from build123d import *

# Parameters (mm, degrees)
ESQUISSE2_W             = 7.209705372
ESQUISSE2_H             = 2.76140959
ENL_V_MAT_EXTRU_1_DEPTH = 7


with BuildPart() as part:
    # Esquisse1 → Révolution1 (revolve)
    with BuildSketch(Plane.XY, mode=Mode.PRIVATE) as r_volution1_sk:
        Polygon((0, 0), (0, 2), (1, 3), (29.26, 3), (29.26, 2.5), (30, 2.5), (30, 3), (44, 3), (45, 2), (45, 0), align=None)
    revolve(r_volution1_sk.sketch.rotate(Axis((-55.939428076, 0, 0), (1, 0, 0)), 90), axis=Axis((-55.939428076, 0, 0), (1, 0, 0)))  # turned: the seam where the file's is

    # Esquisse2 → Enlèv. mat.-Extru.1 (cut)
    with BuildSketch(Plane(origin=(45, 0, 0), x_dir=(0, 0, -1), z_dir=(1, 0, 0))):
        with Locations((-0.271519353, 2.880704795)):
            Rectangle(ESQUISSE2_W, ESQUISSE2_H)
    extrude(amount=-ENL_V_MAT_EXTRU_1_DEPTH, mode=Mode.SUBTRACT)


solid = part.part
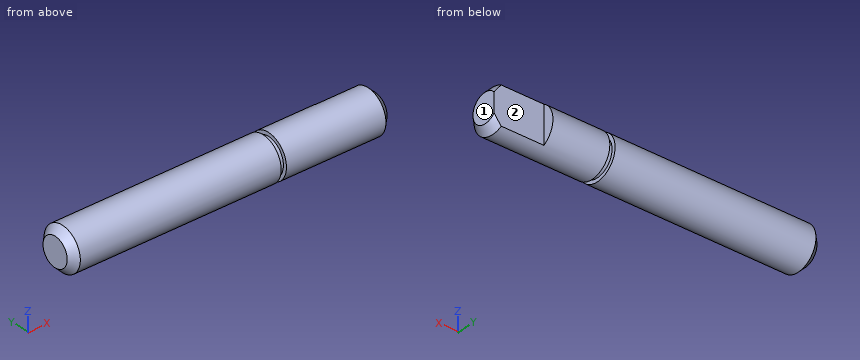
Build history of the part. All positions in model axes, mm. Face numbers are marked on the shaded views. A direction names the side the tool comes from. Round coordinates to 2 decimals unless told otherwise and drop trailing zeros. Loops run counter-clockwise (first coordinate to the right, second up) from the corner with the lowest first, then second, coordinate; pieces in that order, holes last. Notation, with made-up numbers: (69, 84) -> (94, 84) arc R24 cw to (94, 117) -> close; hole circle Ø6 at (62, -25). An arc over 180 degrees is marked (long way). Answer in a Markdown table with one row per item.
Item 1: Which spindle directions (+Z, -Z, +X, -X, +Y, -Y) get a long thin tool onto all of the face, cutting with end or side? Do the marked faces 1 and 2. Say none if no direction does.
Answers below:
| item | result |
|---|---|
| face 1 | +Z, -Z, +X, +Y, -Y |
| face 2 | +Z, -Z, +X, +Y |
Item 2: Saw through at A-A (z = 0). Write the cut outline in (x, y), and give its area (3 significant figures).
Answers below:
| item | result |
|---|---|
| outline | (0, -2) -> (1, -3) -> (29.26, -3) -> (29.26, -2.5) -> (30, -2.5) -> (30, -3) -> (44, -3) -> (45, -2) -> (45, 1.5) -> (38, 1.5) -> (38, 3) -> (30, 3) -> (30, 2.5) -> (29.26, 2.5) -> (29.26, 3) -> (1, 3) -> (0, 2) -> close |
| area | 257 mm² |
Item 3: Pin check, flat tips, straight feed: pin 1 (1.6 mm diameter, centred on x = 41.5, z = -0.5, fed in from +Y); pin 2 (2 mm diameter, centred on x = 37.5, z = -2.5, fed in from +Y). Stop position of each tip, or through.
Answers below:
| item | result |
|---|---|
| pin 1 | stops at y = 1.5 |
| pin 2 | stops at y = 2.6 |
Item 4: Saw through at B-B (x = 33). Write the cut outline in (y, z).
Answers below:
| item | result |
|---|---|
| outline | circle Ø6 at (0, 0) |
Item 5: Drill centre lines: L1, parallel to Y at x = 29.5, z = -1.5; L2, parallel to Z at x = 26, y = 0.2; L3, parallel to X at y = -2.7, z = 0.8. Where is each one in solid material? Low to high. Write a range as [from, to].
Answers below:
| item | result |
|---|---|
| L1 | y = [-2, 2] |
| L2 | z = [-2.99, 2.99] |
| L3 | x = [0.82, 29.26], [30, 44.18] |
